Model file for the job. Use its own axes, mm. A direction names the side the tool comes from. Round coordinates to 2 decimals unless told otherwise and drop trailing zeros. Use a Markdown table: item, result. Add a question column.
Item 1: Tool access for faces 4 (the flat face through (-4, 12.5, 10)), 5 (the flat face through (13, 5, 0)), 6 (the flat face through (12.5, -4, 10)): list every direction of +Z, -Z, +X, -X, +Y, -Y with a clear straight run to the whole face (end or side of a thin tool).
Item 2: Wall check: L1, parallel to X at y = 4.5, z = 24.5; L2, parallel to Y at x = 11, z = 17; L3, parallel to X at y = 27.5, z = 35. Give the ranges that are in metal, low to high. Write a range as from..to.
Item 3: Pin check, flat tips, straight feed: P1, Ø5.5, axis at x = 120, y = 120, coming from the -Z side; P2, Ø13.5, axis at x = 0.5, y = 2, coming from the -Z side; P3, Ø3, axis at y = 1, z = 9, coming from the -X side. Stop position of each tip, or through.
Item 4: Two-plate mould, pull along Y, no slides. Class faces 1 (the cylindrical face through (109.812, 96.091, 375.584)), 2 (the flat face through (-12, -7.5, 10)), 3 (the flat face through (124, 116, 410)): +Y half, -Y half, draft (parallel to the pull), parting line (faces both ways), or undercut.
```python
from build123d import *

# Parameters (mm, degrees)
F0_W      = 40
F0_H      = 40
F2_W      = 40
F2_H      = 40
F4_R      = 3
F5_DEPTH  = 12
F6_R      = 3
F7_DEPTH  = 12
F8_R      = 3
F9_DEPTH  = 12
F11_W     = 20
F11_H     = 20
F12_DEPTH = 32.5
F14_W     = 20
F14_H     = 20
F15_DEPTH = 32.5
F16_R     = 3
F17_DEPTH = 4
F18_R     = 3
F19_DEPTH = 4


with BuildPart() as f3:
    # F0 (on Top) → F3 section 0
    with BuildSketch(Plane.XY):
        Rectangle(F0_W, F0_H)
    # F2 (on offset) → F3 section 1
    with BuildSketch(Plane.XY.offset(410)):
        with Locations((120, 120)):
            Rectangle(F2_W, F2_H)
    loft()

    # F4 (on face) → F5 (cut)
    with BuildSketch(Plane(origin=(-18.4219178082, 0, 5.3917808219), x_dir=(0, -1, 0), z_dir=(-0.959737407, 0, 0.2808987533))):
        with Locations((-112.0100207019, 390.3822122005)):
            Circle(F4_R)
    extrude(amount=-F5_DEPTH, mode=Mode.SUBTRACT)

    # F6 (on face) → F7 (cut)
    with BuildSketch(Plane(origin=(0, -18.4219178082, 5.3917808219), x_dir=(1, 0, 0), z_dir=(0, -0.959737407, 0.2808987533))):
        with Locations((110.461897094, 390.3822122005)):
            Circle(F6_R)
    extrude(amount=-F7_DEPTH, mode=Mode.SUBTRACT)

    # F8 (on face) → F9 (cut)
    with BuildSketch(Plane.XY.offset(410)):
        with Locations((120, 120)):
            Circle(F8_R)
    extrude(amount=-F9_DEPTH, mode=Mode.SUBTRACT)

    # F11 (on offset) → F12 (cut)
    with BuildSketch(Plane.YZ.offset(-20)):
        with Locations((2.5, 10)):
            Rectangle(F11_W, F11_H)
    extrude(amount=F12_DEPTH, mode=Mode.SUBTRACT)

    # F14 (on offset) → F15 (cut)
    with BuildSketch(Plane.XZ.offset(20)):
        with Locations((2.5, 10)):
            Rectangle(F14_W, F14_H)
    extrude(amount=-F15_DEPTH, mode=Mode.SUBTRACT)

    # F16 (on face) → F17 (cut)
    with BuildSketch(Plane.XZ.offset(-12.5)):
        with Locations((2.5, 10)):
            Circle(F16_R)
    extrude(amount=-F17_DEPTH, mode=Mode.SUBTRACT)

    # F18 (on face) → F19 (cut)
    with BuildSketch(Plane(origin=(12.5, 0, 0), x_dir=(0, -1, 0), z_dir=(-1, 0, 0))):
        with Locations((-2.5, 10)):
            Circle(F18_R)
    extrude(amount=-F19_DEPTH, mode=Mode.SUBTRACT)


solid = f3.part
```
Entries:
| question | item | result |
|---|---|---|
| 1 | face 4 | -Z, -X |
| 1 | face 5 | -Z, +X, -X, +Y, -Y |
| 1 | face 6 | -Z, -Y |
| 2 | L1 | -12.83..27.17 |
| 2 | L2 | 12.5..24.98 |
| 2 | L3 | -9.76..30.24 |
| 3 | P1 | z = 335.02 |
| 3 | P2 | z = 20 |
| 3 | P3 | x = 12.5 |
| 4 | face 1 | undercut |
| 4 | face 2 | undercut |
| 4 | face 3 | draft |
